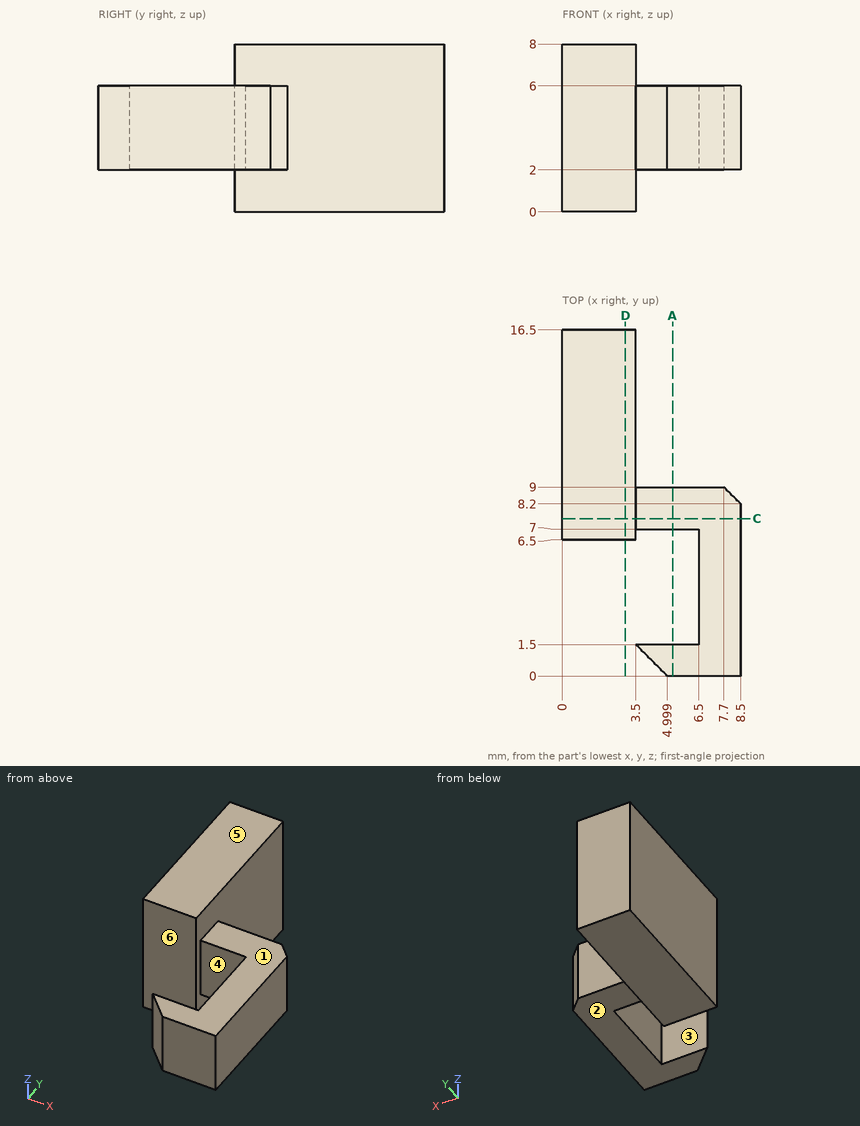
Print and shaded views of the part. All mm, measured from the part's lowest x, y and z. A direction names the side the tool comes from. Give positions to 0.01 mm unless a question says otherwise; leave off trailing zeros. Loops run counter-clockwise (first coordinate to the right, second up) from the corner with the lowest first, then second, coordinate; pieces in that order, holes last. Notation, with made-up numbers: (37, 15) -> (41, 15) arc R26 cw to (41, 31) -> close; hole circle Ø11 at (72.5, 15.25). An arc over 180 degrees is marked (long way). Answer in a Markdown table with one row per item.
Item 1: Tool access for the marked faces 1, 2 and 3: list every direction of +Z, -Z, +X, -X, +Y, -Y with a clear straight run to the whole face (end or side of a thin tool).
Findings below:
| item | result |
|---|---|
| face 1 | +Z, +X, +Y, -Y |
| face 2 | -Z, +X, +Y, -Y |
| face 3 | +Z, -Z, -X |
Item 2: Slice it at D-D on x = 3. Write the cut outline in (y, z).
Findings below:
| item | result |
|---|---|
| outline | (6.5, 0) -> (16.5, 0) -> (16.5, 8) -> (6.5, 8) -> close |
Item 3: Slice it at A-A on x = 5.25. Write the cut outline in (y, z).
Findings below:
| item | result |
|---|---|
| outline | (0, 2) -> (1.5, 2) -> (1.5, 6) -> (0, 6) -> close; (7, 2) -> (9, 2) -> (9, 6) -> (7, 6) -> close |
Item 4: Probe line 1 along Y through (x, z) = (6, 2.5); line 2 along X through (y, z) = (5, 5); line 3 along X through (y, z) = (9.75, 7.25). List the from-to ranges inside material, lowest first. Write a range as [from, to].
Findings below:
| item | result |
|---|---|
| line 1 | y = [0, 1.5], [7, 9] |
| line 2 | x = [6.5, 8.5] |
| line 3 | x = [0, 3.5] |
Item 5: Mould opens along Y. For the marked faces 4, 5 and 6 say: pulls with the +Y half, pulls with the -Y half, needs draft (parallel to the pull), parting line crosses it, or undercut.
Findings below:
| item | result |
|---|---|
| face 4 | undercut |
| face 5 | needs draft |
| face 6 | pulls with the -Y half |
Item 6: Flat gauge pins, fed straight in: P1, Ø1.5, axis at x = 7, y = 6, coming from the +Z side; P2, Ø4, axis at y = 10.5, z = 3, coming from the +X side; P3, Ø1.8, axis at x = 2.5, z = 3, coming from the -Y side. Where does each tip first touch, or does it go through?
Findings below:
| item | result |
|---|---|
| P1 | stops at z = 6 |
| P2 | stops at x = 8.2 |
| P3 | stops at y = 6.5 |
Item 7: Slice it at C-C on y = 7.5. Write the cut outline in (x, z).
Findings below:
| item | result |
|---|---|
| outline | (0, 0) -> (3.5, 0) -> (3.5, 2) -> (8.5, 2) -> (8.5, 6) -> (3.5, 6) -> (3.5, 8) -> (0, 8) -> close |
